Autodesk Inventor part; units mm, degrees
ref_plane "YZ Plane" through (0, 0, 0) normal (1, 0, 0) x (0, 1, 0)
ref_plane "XZ Plane" through (0, 0, 0) normal (0, 1, 0) x (-1, 0, 0)
ref_plane "XY Plane" through (0, 0, 0) normal (0, 0, 1) x (1, 0, 0)
sketch "Sketch1" plane through (0, 0, 0) normal (0, 1, 0) x (-1, 0, 0)
  line L0 (0, 0) -> (25, 0)
  line L1 (25, 0) -> (25, -25)
  line L2 (25, -25) -> (20, -25)
  line L3 (20, -25) -> (20, -5)
  line L4 (20, -5) -> (0, -5)
  line L5 (0, -5) -> (0, 0)
  dimension "d0" = 5
  dimension "d1" = 25
  dimension "d2" = 25
extrude "Extrusion1" add sketch "Sketch1" along normal mid plane 10
sketch "Sketch2" plane through (-20, -5, -25) normal (1, 0, 0) x (0, 0, -1)
  circle A0 centre (-5, 5) radius 2
  line L0 (-25, 0) -> (-25, 10)
  line L1 (-20, 10) -> (0, 10)
  line L2 (0, 0) -> (0, 10)
  point P0 (-25, 5)
  point P1 (-25, 5)
  dimension "d5" = 4
  dimension "d9" = 5
extrude "Extrusion2" cut sketch "Sketch2" against normal through all
sketch "Sketch3" plane through (0, 5, -5) normal (0, 0, -1) x (-1, 0, 0)
  circle A0 centre (5, -5) radius 1.75
  line L0 (0, 0) -> (0, -10)
  line L1 (0, 0) -> (20, 0)
  point P0 (0, -5)
  point P1 (0, -5)
  point P2 (0, -5)
  dimension "d8" = 3.5
  dimension "d11" = 5
extrude "Extrusion3" cut sketch "Sketch3" against normal blind 10
chamfer "Chamfer1" distance 2 angle 45 2 edges at (-25, 0, 0) (-20, 0, -5)
properties part number "L connection"
Geometry check sheet. Reference: the model listing, model coordinates, mm. A direction names the side the tool comes from. Round coordinates to 2 decimals unless told otherwise and drop trailing zeros. Order: outer loops, then holes, each group sorted by start corner. A loop starts at its lowest first (then second) coordinate and runs counter-clockwise, first axis right, second up. Notation, with made-up numbers: M 18,-23.75 L 40,-23.75 A24 cw 40,-8.75 Z; hole C 31,-1 d4. An arc over 180 degrees is marked long. Answer in a Markdown table with one row per item. Add a question column.
Item 1: Sectioned sample at A-A, the plane x = -5. Enter the section's corners in (y, z).
Item 2: Material ranges on L1, parallel to Y at x = -5, z = -2.15; L2, parallel to Z at x = -11.25, y = 3; L3, parallel to X at y = 1.75, z = -22.5, recorded low to high. Write a range as [from, to].
Item 3: Sectioned sample at D-D, the plane y = -2.5. Enter the section's corners in (x, z).
Item 4: Sectioned sample at C-C, the plane z = -20. Enter the section's corners in (x, y), plus the area to 3 significant figures.
Item 5: Sectioned sample at B-B, the plane y = 0. Enter the section's corners in (x, z).
Item 6: Set-up check for faces 5 (the face through (-9, 0, -5)), 6 (the face through (-25, 0, -13)): record each of +Z, -Z, +X, -X, +Y, -Y from which the full face is reachable in a straight line by a thin tool's end or side.
Item 7: Draft check along Z on faces 1 (the face through (-22.5, -1.2, -18.4)), 2 (the face through (0, 0, -3)), 3 (the face through (-24, 0, -1)), 4 (the face through (-23, 0, -25)). Enter one of: released by +Z, released by -Z, zero draft, split by the parting line, or undercut.
Item 8: Depth check by flat-ended pin: pin 1 Ø4 at (x, y) = (-5, 0) entering from -Z; pin 2 Ø5 at (y, z) = (2, -16.5) entering from +X. Enter the tip coordinate at first touch or a pass-through.
Filled in:
| question | item | result |
|---|---|---|
| 1 | outline | M -5,-5 L -1.75,-5 L -1.75,0 L -5,0 Z; M 1.75,-5 L 5,-5 L 5,0 L 1.75,0 Z |
| 2 | L1 | y = [-5, -1.75], [1.75, 5] |
| 2 | L2 | z = [-5, 0] |
| 2 | L3 | x = [-25, -20] |
| 3 | outline | M -25,-25 L -20,-25 L -20,-7 L -18,-5 L 0,-5 L 0,0 L -23,0 L -25,-2 Z |
| 4 | outline | M -25,-5 L -20,-5 L -20,-2 L -25,-2 Z; M -25,2 L -20,2 L -20,5 L -25,5 Z |
| 4 | area | 30.0 mm² |
| 5 | outline | M -25,-25 L -20,-25 L -20,-22 L -25,-22 Z; M -25,-18 L -20,-18 L -20,-7 L -18,-5 L -6.75,-5 L -6.75,0 L -23,0 L -25,-2 Z; M -3.25,-5 L 0,-5 L 0,0 L -3.25,0 Z |
| 6 | face 5 | -Z, +X, +Y, -Y |
| 6 | face 6 | +Z, -Z, -X, +Y, -Y |
| 7 | face 1 | undercut |
| 7 | face 2 | zero draft |
| 7 | face 3 | released by +Z |
| 7 | face 4 | released by -Z |
| 8 | pin 1 | stops at z = -5 |
| 8 | pin 2 | stops at x = -20 |
